```python
from build123d import *

# Parameters (mm, degrees)
CUT_EXTRUDE3_DEPTH = 10


with BuildPart() as part:
    # Sketch1 → Revolve2 (revolve)
    with BuildSketch(Plane.XY, mode=Mode.PRIVATE) as revolve2_sk:
        Polygon((10, 0), (20, 0), (20, 3), (19.5, 3), (19.5, 7.75), (17.343396893, 7.75), (17.343396893, 9.25), (18.843396893, 9.25), (18.843396893, 12.5), (10, 12.5), align=None)
    revolve(revolve2_sk.sketch.rotate(Axis((0, 0, 0), (0, 1, 0)), 90), axis=Axis((0, 0, 0), (0, 1, 0)))

    # Sketch2 → Cut-Extrude3 (cut)
    with BuildSketch(Plane(origin=(0, 12.5, 0), x_dir=(1, 0, 0), z_dir=(0, 1, 0))):
        with BuildLine():
            ThreePointArc((13.776115673, 12.856603107), (0, 18.843396893), (-13.776115673, 12.856603107))
            Line((-13.776115673, 12.856603107), (13.776115673, 12.856603107))
        make_face()
    extrude(amount=-CUT_EXTRUDE3_DEPTH, mode=Mode.SUBTRACT)


solid = part.part
```
Source: CAD feature listing. Evaluate the final solid. Frame: model axes, mm. A direction names the side the tool comes from. Give positions to 0.01 mm unless a question says otherwise; leave off trailing zeros. Loops run counter-clockwise (first coordinate to the right, second up) from the corner with the lowest first, then second, coordinate; pieces in that order, holes last. Notation, with made-up numbers: (-17.5, 54.5) -> (17.5, 54.5) arc R15 ccw to (17.5, 82.5) -> close; hole circle Ø8 at (15.25, -4). An arc over 180 degrees is marked (long way). Use a Markdown table: item, result. Add a question column.
(1) Section query A-A (x = 0). Output: boundary loops of the cut face in (y, z), then the cut area to 3 significant figures.
(2) Pull-direction query (Z, two-part tool) for faces 1 (the face through (0, 2.5, -15)), 2 (the face through (-19.334, 5.408, 2.539)), 3 (the face through (-9, 0, -5)); classes: +Z half, -Z half, draft (parallel to the pull), parting line (faces both ways), or undercut.
(3) Section query C-C (y = 10.75). Output: boundary loops of the cut face in (x, z).
(4) Section query B-B (z = 0). Output: boundary loops of the cut face in (x, y), then the cut area to 3 significant figures.
(5) Access query for faces 4 (the face through (4.4, 3, -19.2)), 5 (the face through (-0.3, 12.5, 10.3)), 6 (the face through (4.1, 9.25, 17.01)). Directions: +Z, -Z, +X, -X, +Y, -Y. A direction counts if a zero-diameter tool reaches every point of the face in a straight line with its end or side. Return the directions, or none.
(6) Section query D-D (z = -11). Output: boundary loops of the cut face in (x, y), then the cut area to 3 significant figures.
(7) First-contact query: pin 1 Ø1.5 at (x, z) = (-7, 10.5) entering from -Y; pin 2 Ø5 at (x, y) = (2, 6.5) entering from -Z; pin 3 Ø12 at (x, z) = (0, 0) entering from -Y; pin 4 Ø2 at (y, z) = (8.5, -1.5) entering from -X. Flat tips, straight axial feed; report the tip coordinate or a pass-through.
(8) Ray query, line 1 (Z direction, x = 0.5, y = 4.25); line 2 (X direction, y = 5.5, z = 0); line 3 (X direction, y = 8.25, z = 0). Return the intervals inside material, ascending.
Checked values:
| question | item | result |
|---|---|---|
| 1 | outline | (0, -20) -> (3, -20) -> (3, -19.5) -> (7.75, -19.5) -> (7.75, -18.84) -> (2.5, -18.84) -> (2.5, -12.86) -> (12.5, -12.86) -> (12.5, -10) -> (0, -10) -> close; (0, 10) -> (12.5, 10) -> (12.5, 18.84) -> (9.25, 18.84) -> (9.25, 17.34) -> (7.75, 17.34) -> (7.75, 19.5) -> (3, 19.5) -> (3, 20) -> (0, 20) -> close |
| 1 | area | 172 mm^2 |
| 2 | face 1 | undercut |
| 2 | face 2 | parting line |
| 2 | face 3 | draft |
| 3 | outline | (-13.78, -12.86) -> (13.78, -12.86) arc R18.84 ccw (long way) to start; hole circle Ø20 at (0, 0) |
| 4 | outline | (-20, 0) -> (-10, 0) -> (-10, 12.5) -> (-18.84, 12.5) -> (-18.84, 9.25) -> (-17.34, 9.25) -> (-17.34, 7.75) -> (-19.5, 7.75) -> (-19.5, 3) -> (-20, 3) -> close; (10, 0) -> (20, 0) -> (20, 3) -> (19.5, 3) -> (19.5, 7.75) -> (17.34, 7.75) -> (17.34, 9.25) -> (18.84, 9.25) -> (18.84, 12.5) -> (10, 12.5) -> close |
| 4 | area | 230 mm^2 |
| 5 | face 4 | +Y |
| 5 | face 5 | +Z, -Z, +X, -X, +Y |
| 5 | face 6 | none |
| 6 | outline | (-16.7, 0) -> (16.7, 0) -> (16.7, 3) -> (16.1, 3) -> (16.1, 7.75) -> (13.41, 7.75) -> (13.41, 9.25) -> (15.3, 9.25) -> (15.3, 12.5) -> (-15.3, 12.5) -> (-15.3, 9.25) -> (-13.41, 9.25) -> (-13.41, 7.75) -> (-16.1, 7.75) -> (-16.1, 3) -> (-16.7, 3) -> close |
| 6 | area | 393 mm^2 |
| 7 | pin 1 | y = 0 |
| 7 | pin 2 | z = -19.5 |
| 7 | pin 3 | through |
| 7 | pin 4 | x = -19.48 |
| 8 | line 1 | -19.49 to -18.84, -12.86 to -9.99, 9.99 to 19.49 |
| 8 | line 2 | -19.5 to -10, 10 to 19.5 |
| 8 | line 3 | -17.34 to -10, 10 to 17.34 |
